Geometry check sheet. Reference: the model listing, model coordinates, mm. Round coordinates to 2 decimals unless told otherwise and drop trailing zeros. Loops run counter-clockwise (first coordinate to the right, second up) from the corner with the lowest first, then second, coordinate; pieces in that order, holes last. Notation, with made-up numbers: (12, 30) - (46, 30) arc R16 ccw to (46, 37) - close; hole circle Ø2 at (62.5, 53). An arc over 180 degrees is marked (long way). Write item = value, one per line.
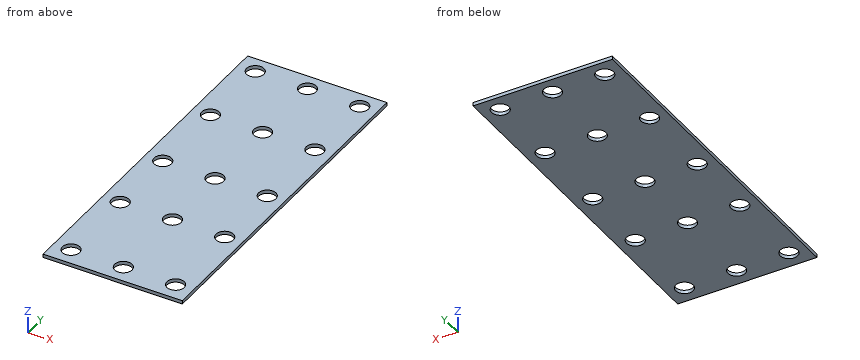
```python
from build123d import *

# Parameters (mm, degrees)
F0_W       = 50.8
F0_H       = 127
F1_DEPTH   = 1.27
F3_D       = 6.35
F3_ON_F0_D = 6.35


with BuildPart() as f1:
    # F0 (on Top) → F1 (new body)
    with BuildSketch(Plane.XY):
        Rectangle(F0_W, F0_H)
    extrude(amount=F1_DEPTH)

    # F3 (through all)
    with Locations(Plane(origin=(0, 0, 0), x_dir=(1, 0, 0), z_dir=(0, 0, -1))):
        with Locations((-19.05, -57.4053688833), (0, -57.4053688833), (19.05, -57.4053688833), (19.05, -29.5683733465), (0, -29.5683733465), (-19.05, -29.5683733465), (-19.05, 0), (19.05, 0), (19.05, 26.3971900072), (0, 56.8946311167), (0, 26.3971900072), (-19.05, 26.3971900072), (-19.05, 56.8946311167), (19.05, 56.8946311167)):
            Hole(F3_D / 2)

    # F3 on F0 (through all)
    with Locations(Plane(origin=(0, 0, 0), x_dir=(1, 0, 0), z_dir=(0, 0, -1))):
        with Locations((0, 0)):
            Hole(F3_ON_F0_D / 2)


solid = f1.part
```
(1) Section check A-A (y = 0). Enter the section's corners in (x, z) (3 decimals), then the cut area to 3 significant figures.
Answers follow:
outline = (-25.4, 0) - (-22.225, 0) - (-22.225, 1.27) - (-25.4, 1.27) - close; (-15.875, 0) - (-3.175, 0) - (-3.175, 1.27) - (-15.875, 1.27) - close; (3.175, 0) - (15.875, 0) - (15.875, 1.27) - (3.175, 1.27) - close; (22.225, 0) - (25.4, 0) - (25.4, 1.27) - (22.225, 1.27) - close
area = 40.3 mm²
(2) Scan lines: L1, parallel to Y at x = 19.05, z = 0.5 (3 decimals); L2, parallel to X at y = -26, z = 0.55; L3, parallel to X at y = 1, z = 0.25. Record each from-to range of solid material in increasing order. Write a range as [from, to].
Answers follow:
L1 = [-63.5, -60.07], [-53.72, -29.572], [-23.222, -3.175], [3.175, 26.393], [32.743, 54.23], [60.58, 63.5]
L2 = [-25.4, -22.2], [-15.9, -3.15], [3.15, 15.9], [22.2, 25.4]
L3 = [-25.4, -22.06], [-16.04, -3.01], [3.01, 16.04], [22.06, 25.4]
(3) Section check C-C (z = 0.2). State how many separate pieces and enclosed holes the cut face has, then the cut area to 3 significant figures.
Answers follow:
separate_pieces = 1
enclosed_holes = 15
area = 5,980 mm²
(4) Gauge pin test, flat end, axial feed: pin 1 (5 mm diameter, centred on x = 19.05, y = -56.89, fed in from +Z) (3 decimals). Record the tip position at first contact, or that the pin passes through.
Answers follow:
pin_1 = through
(5) Section check B-B (x = -19.05). Enter the section's corners in (y, z) (3 decimals).
Answers follow:
outline = (-63.5, 0) - (-60.07, 0) - (-60.07, 1.27) - (-63.5, 1.27) - close; (-53.72, 0) - (-29.572, 0) - (-29.572, 1.27) - (-53.72, 1.27) - close; (-23.222, 0) - (-3.175, 0) - (-3.175, 1.27) - (-23.222, 1.27) - close; (3.175, 0) - (26.393, 0) - (26.393, 1.27) - (3.175, 1.27) - close; (32.743, 0) - (54.23, 0) - (54.23, 1.27) - (32.743, 1.27) - close; (60.58, 0) - (63.5, 0) - (63.5, 1.27) - (60.58, 1.27) - close
